Model file for the job. Use its own axes, mm. Coordinates: 2 decimals unless noted, no trailing zeros. Loops run counter-clockwise (first coordinate to the right, second up) from the corner with the lowest first, then second, coordinate; pieces in that order, holes last. Notation, with made-up numbers: (73.5, 6) -> (92.5, 6) arc R17 ccw to (92.5, 11) -> close; hole circle Ø11 at (38.25, 0.25). An arc over 180 degrees is marked (long way). Use one line per item in the form item = value.
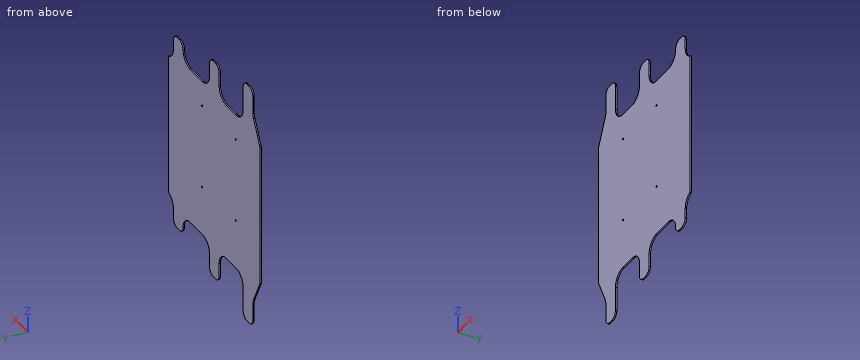
```python
from build123d import *

# Parameters (mm, degrees)
SKETCH1_W             = 380
SKETCH1_H             = 326
BOSS_EXTRUDE1_DEPTH   = 3
SKETCH2_R             = 2
PCB_PLATE_HOLES_DEPTH = 3
BOSS_EXTRUDE2_DEPTH   = 3
FILLET1_R             = 30
FILLET2_R             = 15


# Some blends are built 0.0001 mm under size
with BuildPart() as part:
    # Sketch1 → Boss-Extrude1 (new body)
    with BuildSketch(Plane(origin=(0, 0, 0), x_dir=(1, 0, 0), z_dir=(0, 1, 0))):
        Rectangle(SKETCH1_W, SKETCH1_H)
    extrude(amount=BOSS_EXTRUDE1_DEPTH)

    # Sketch2 → PCB Plate Holes (cut)
    with BuildSketch(Plane(origin=(0, 3, 0), x_dir=(1, 0, 0), z_dir=(0, 1, 0))):
        with Locations(Location((51, 70, 0), (0, 0, 270))):
            Circle(SKETCH2_R)
        with Locations(Location((-89, 70, 0), (0, 0, 270))):
            Circle(SKETCH2_R)
        with Locations(Location((51, -124, 0), (0, 0, 270))):
            Circle(SKETCH2_R)
        with Locations(Location((-89, -124, 0), (0, 0, 270))):
            Circle(SKETCH2_R)
    extrude(amount=-PCB_PLATE_HOLES_DEPTH, mode=Mode.SUBTRACT)

    # Sketch3 → Boss-Extrude2 (add)
    with BuildSketch(Plane(origin=(0, 3, 0), x_dir=(1, 0, 0), z_dir=(0, 1, 0))):
        Polygon((170, 163), (170, 228), (130, 228), (130, 183), (20, 183), (20, 258), (-20, 258), (-20, 183), (-120, 183), (-120, 283), (-160, 283), (-160, 223), (-190, 163), align=None)
        Polygon((170, -228), (170, -163), (-190, -163), (-160, -223), (-160, -283), (-120, -283), (-120, -183), (-20, -183), (-20, -258), (20, -258), (20, -183), (130, -183), (130, -228), align=None)
    extrude(amount=-BOSS_EXTRUDE2_DEPTH)

    # Fillet1
    # the kernel refuses this fillet: 30 mm, written as the material it adds along each edge
    with BuildSketch(Plane(origin=(130, 3, -183), x_dir=(0, 0, -1), z_dir=(0, -1, 0)), Plane(origin=(20, 3, -183), x_dir=(1, 0, 0), z_dir=(0, -1, 0)), Plane(origin=(-20, 3, -183), x_dir=(0, 0, -1), z_dir=(0, -1, 0)), Plane(origin=(-120, 3, -183), x_dir=(1, 0, 0), z_dir=(0, -1, 0)), Plane(origin=(20, 3, 183), x_dir=(0, 0, 1), z_dir=(0, -1, 0)), Plane(origin=(130, 3, 183), x_dir=(-1, 0, 0), z_dir=(0, -1, 0)), Plane(origin=(-20, 3, 183), x_dir=(-1, 0, 0), z_dir=(0, -1, 0)), Plane(origin=(-120, 3, 183), x_dir=(0, 0, 1), z_dir=(0, -1, 0))) as fillet1_piece_1:
        with BuildLine():
            CenterArc((FILLET1_R, -FILLET1_R), FILLET1_R, 90, 90)
            Line((0, -FILLET1_R), (-FILLET1_R * 0.02, -FILLET1_R))
            Line((-FILLET1_R * 0.02, -FILLET1_R), (-FILLET1_R * 0.02, FILLET1_R * 0.02))
            Line((-FILLET1_R * 0.02, FILLET1_R * 0.02), (FILLET1_R, FILLET1_R * 0.02))
            Line((FILLET1_R, FILLET1_R * 0.02), (FILLET1_R, 0))
        make_face()
    extrude(amount=3)
    with BuildSketch(Plane(origin=(170, 3, -163), x_dir=(1, 0, 0), z_dir=(0, -1, 0))) as fillet1_piece_2:
        with BuildLine():
            CenterArc((30, -28.284271247), FILLET1_R, 109.471220634, 70.528779366)
            Line((0, -28.284271247), (-0.6, -28.284271247))
            Line((-0.6, -28.284271247), (-0.6, 0))
            Line((-0.6, 0), (0, 0.6))
            ThreePointArc((0, 0.6), (10, 0.6), (19.8, 0.565685425))
            Line((19.8, 0.565685425), (20, 0))
        make_face()
    extrude(amount=3)
    with BuildSketch(Plane(origin=(170, 3, 163), x_dir=(1, 0, 0), z_dir=(0, -1, 0))) as fillet1_piece_3:
        with BuildLine():
            CenterArc((30, 28.284271247), FILLET1_R, 180, 70.528779366)
            Line((0, 28.284271247), (-0.6, 28.284271247))
            Line((-0.6, 28.284271247), (-0.6, 0))
            Line((-0.6, 0), (0, -0.6))
            ThreePointArc((0, -0.6), (10, -0.6), (19.8, -0.565685425))
            Line((19.8, -0.565685425), (20, 0))
        make_face()
    extrude(amount=3)
    with BuildSketch(Plane(origin=(-160, 3, -223), x_dir=(-0.44721359549995476, 0, 0.8944271909999175), z_dir=(0, -1, 0))) as fillet1_piece_4:
        with BuildLine():
            CenterArc((FILLET1_R * 0.2360679775, FILLET1_R), FILLET1_R, 243.434948823, 26.565051177)
            Line((-FILLET1_R * 0.211145618, FILLET1_R * 0.105572809), (-FILLET1_R * 0.22008988991, FILLET1_R * 0.0876842651801))
            Line((-FILLET1_R * 0.22008988991, FILLET1_R * 0.0876842651801), (-FILLET1_R * 0.00472135955, -FILLET1_R * 0.02))
            Line((-FILLET1_R * 0.00472135955, -FILLET1_R * 0.02), (FILLET1_R * 0.2360679775, -FILLET1_R * 0.02))
            Line((FILLET1_R * 0.2360679775, -FILLET1_R * 0.02), (FILLET1_R * 0.2360679775, 0))
        make_face()
    extrude(amount=3)
    with BuildSketch(Plane(origin=(-160, 3, 223), x_dir=(-0.4472135954999563, 0, -0.8944271909999166), z_dir=(0, -1, 0))) as fillet1_piece_5:
        with BuildLine():
            CenterArc((FILLET1_R * 0.2360679775, -FILLET1_R), FILLET1_R, 90, 26.565051177)
            Line((-FILLET1_R * 0.211145618, -FILLET1_R * 0.105572809), (-FILLET1_R * 0.22008988991, -FILLET1_R * 0.0876842651801))
            Line((-FILLET1_R * 0.22008988991, -FILLET1_R * 0.0876842651801), (-FILLET1_R * 0.00472135955, FILLET1_R * 0.02))
            Line((-FILLET1_R * 0.00472135955, FILLET1_R * 0.02), (FILLET1_R * 0.2360679775, FILLET1_R * 0.02))
            Line((FILLET1_R * 0.2360679775, FILLET1_R * 0.02), (FILLET1_R * 0.2360679775, 0))
        make_face()
    extrude(amount=3)

    # Fillet2
    fillet2_edges = [part.edges().sort_by_distance(p)[0] for p in [
        (170, 1.5, 228),
        (130, 1.5, 228),
        (20, 1.5, 258),
        (-120, 1.5, 283),
        (-20, 1.5, 258),
        (170, 1.5, -228),
        (130, 1.5, -228),
        (20, 1.5, -258),
        (-20, 1.5, -258),
        (-120, 1.5, -283),
        (-160, 1.5, -283),
        (-160, 1.5, 283),
    ]]
    fillet(fillet2_edges, radius=FILLET2_R - 0.0001)  # a hair under: the kernel refuses the full size


solid = part.part
```
Q1. Band-saw the part on A-A, the plane x = -78.5. Write the cut outline in (y, z).
Result:
outline = (0, -183) -> (3, -183) -> (3, 183) -> (0, 183) -> close
Q2. Band-saw the part on C-C, the plane x = 106. Write the cut outline in (y, z).
Result:
outline = (0, -183.61) -> (3, -183.61) -> (3, 183.61) -> (0, 183.61) -> close
Q3. Pin check, flat tips, straight feed: pin 1 Ø0.9 at (y, z) = (1, -235.5) entering from +X; pin 2 Ø0.9 at (x, y) = (69, 1.5) entering from +Z; pin 3 Ø1.5 at (x, y) = (2, 1.5) entering from -Z. Stop position of each tip, or through.
Result:
pin_1 = 20
pin_2 = 183
pin_3 = -258
Q4. Band-saw the part on B-B, the plane y = 0.7. State how many separate pieces and enclosed holes the cut face has, and give its area (3 significant figures).
Result:
separate_pieces = 1
enclosed_holes = 4
area = 158,000 mm2
Q5. Wall check: line 1 along X through (y, z) = (1.7, 124); line 2 along X through (y, z) = (1.1, 213.5); line 3 along Z through (x, y) = (-91.5, 1.6). Give the ranges that are in metal, low to high.
Result:
line_1 = -190 to -91, -87 to 49, 53 to 190
line_2 = -164.75 to -120, -20 to 20, 130.01 to 169.99
line_3 = -183.04 to 183.04
